from build123d import *
from build123d.topology import SkipClean

# Parameters (mm, degrees)
ESQUISSE1_W              = 55
ESQUISSE1_H              = 45
BOSS_EXTRU_1_DEPTH       = 12
ESQUISSE2_R              = 4.25
ENL_V_MAT_EXTRU_1_DEPTH  = 55.085580333
ESQUISSE3_R              = 7.75
ENL_V_MAT_EXTRU_2_DEPTH  = 12.25
ESQUISSE9_W              = 61.062756781
ESQUISSE9_H              = 12.22812859
ESQUISSE9_W_2            = 59.427147224
ESQUISSE9_H_2            = 8.100161614
ENL_V_MAT_EXTRU_7_DEPTH  = 31
SKETCH1_W                = 55
SKETCH1_H                = 36
BOSS_EXTRUDE1_DEPTH      = 5
SKETCH2_R                = 2.1
CUT_EXTRUDE1_DEPTH       = 38.003378224
SKETCH3_R                = 4
CUT_EXTRUDE2_DEPTH       = 10
CUT_EXTRUDE3_DEPTH       = 5
SKETCH5_R                = 2.1
CUT_EXTRUDE4_DEPTH       = 47.864165415
BOSS_EXTRUDE4_START      = 2
SKETCH7_R                = 2.1
BOSS_EXTRUDE4_DEPTH      = 2
SKETCH8_R                = 2.1
BOSS_EXTRUDE5_DEPTH      = 2
SKETCH9_W                = 7
SKETCH9_H                = 3.2
CUT_EXTRUDE6_DEPTH       = 8
SKETCH10_W               = 30
SKETCH10_H               = 15
BOSS_EXTRUDE6_DEPTH      = 90
BOSS_EXTRUDE7_DEPTH      = 5
BOSS_EXTRUDE7_DEPTH_BACK = 5


with BuildPart() as part:
    # Esquisse1 → Boss.-Extru.1 (new body)
    with BuildSketch(Plane.XY):
        Rectangle(ESQUISSE1_W, ESQUISSE1_H)
    extrude(amount=BOSS_EXTRU_1_DEPTH)

    # Esquisse2 → Enl_v. mat.-Extru.1 (cut, through all)
    with BuildSketch(Plane(origin=(0, 22.5, 0), x_dir=(1, 0, 0), z_dir=(0, 1, 0))):
        with Locations((-12.5, -12)):
            Circle(ESQUISSE2_R)
        with Locations((12.5, -12)):
            Circle(ESQUISSE2_R)
    extrude(amount=-ENL_V_MAT_EXTRU_1_DEPTH, mode=Mode.SUBTRACT)

    # Esquisse3 → Enl_v. mat.-Extru.2 (cut, symmetric)
    with BuildSketch(Plane(origin=(0, 0, 0), x_dir=(1, 0, 0), z_dir=(0, 1, 0))):
        with Locations((-12.5, -12)):
            Circle(ESQUISSE3_R)
    enl_v_mat_extru_2 = extrude(amount=ENL_V_MAT_EXTRU_2_DEPTH, both=True, mode=Mode.SUBTRACT)

    # Esquisse9 → Enl_v. mat.-Extru.7 (cut)
    with BuildSketch(Plane.XY.offset(12)):
        with Locations((-0.389430846, -24.114064295)):
            Rectangle(ESQUISSE9_W, ESQUISSE9_H)
        with Locations((1.674552641, 22.050080807)):
            Rectangle(ESQUISSE9_W_2, ESQUISSE9_H_2)
    extrude(amount=-ENL_V_MAT_EXTRU_7_DEPTH, mode=Mode.SUBTRACT)

    # Sketch1 → Boss-Extrude1 (add)
    with BuildSketch(Plane(origin=(0, 0, 0), x_dir=(-1, 0, 0), z_dir=(0, 0, -1))):
        Rectangle(SKETCH1_W, SKETCH1_H)
    extrude(amount=BOSS_EXTRUDE1_DEPTH)

    # Sketch2 → Cut-Extrude1 (cut, through all)
    with BuildSketch(Plane.XY.offset(12)):
        with Locations((-22.5, 13)):
            Circle(SKETCH2_R)
        with Locations(Location((22.5, 13, 0), (0, 0, 180))):
            Circle(SKETCH2_R)
        with Locations((22.5, -13)):
            Circle(SKETCH2_R)
        with Locations(Location((-22.5, -13, 0), (0, 0, 180))):
            Circle(SKETCH2_R)
    extrude(amount=-CUT_EXTRUDE1_DEPTH, mode=Mode.SUBTRACT)

    # Sketch3 → Cut-Extrude2 (cut)
    with BuildSketch(Plane(origin=(0, 0, -5), x_dir=(-1, 0, 0), z_dir=(0, 0, -1))):
        with Locations((-22.5, 13)):
            Circle(SKETCH3_R)
        with Locations((22.5, 13)):
            Circle(SKETCH3_R)
        with Locations((22.5, -13)):
            Circle(SKETCH3_R)
        with Locations((-22.5, -13)):
            Circle(SKETCH3_R)
    extrude(amount=-CUT_EXTRUDE2_DEPTH, mode=Mode.SUBTRACT)

    # Sketch4 → Cut-Extrude3 (cut)
    with BuildSketch(Plane(origin=(0, 0, -5), x_dir=(-1, 0, 0), z_dir=(0, 0, -1))):
        with BuildLine():
            Line((-18.5, 13), (-18.5, 18))
            Line((-18.5, 18), (-27.5, 18))
            Line((-27.5, 18), (-27.5, 9))
            Line((-27.5, 9), (-22.5, 9))
            ThreePointArc((-22.5, 9), (-25.328427125, 15.828427125), (-18.5, 13))
        make_face()
        with BuildLine():
            Line((-22.5, -9), (-27.5, -9))
            Line((-27.5, -9), (-27.5, -18))
            Line((-27.5, -18), (-18.5, -18))
            Line((-18.5, -18), (-18.5, -13))
            ThreePointArc((-18.5, -13), (-25.328427125, -15.828427125), (-22.5, -9))
        make_face()
        with BuildLine():
            Line((27.5, -18), (27.5, -9))
            Line((27.5, -9), (22.5, -9))
            ThreePointArc((22.5, -9), (25.328427125, -15.828427125), (18.5, -13))
            Line((18.5, -13), (18.5, -18))
            Line((18.5, -18), (27.5, -18))
        make_face()
        with BuildLine():
            Line((27.5, 18), (18.5, 18))
            Line((18.5, 18), (18.5, 13))
            ThreePointArc((18.5, 13), (25.328427125, 15.828427125), (22.5, 9))
            Line((22.5, 9), (27.5, 9))
            Line((27.5, 9), (27.5, 18))
        make_face()
    extrude(amount=-CUT_EXTRUDE3_DEPTH, mode=Mode.SUBTRACT)

    # Sketch5 → Cut-Extrude4 (cut, through all)
    with BuildSketch(Plane(origin=(0, 18, 0), x_dir=(1, 0, 0), z_dir=(0, 1, 0))):
        with Locations(Location((-10, 1, 0), (0, 0, 180))):
            Circle(SKETCH5_R)
        with Locations(Location((10, 1, 0), (0, 0, 180))):
            Circle(SKETCH5_R)
    extrude(amount=-CUT_EXTRUDE4_DEPTH, mode=Mode.SUBTRACT)

    # Sketch7 → Boss-Extrude4 (add)
    with SkipClean():  # the faces are left unmerged after this step: merging them gives an invalid solid
        with BuildSketch(Plane(origin=(0, 18, 0), x_dir=(1, 0, 0), z_dir=(0, 1, 0)).offset(BOSS_EXTRUDE4_START)):
            with BuildLine():
                Line((18.5, 5), (-18.5, 5))
                Line((-18.5, 5), (-18.5, 0))
                Line((-18.5, 0), (-27.5, 0))
                Line((-27.5, 0), (-27.5, -12))
                Line((-27.5, -12), (-16.75, -12))
                ThreePointArc((-16.75, -12), (-12.5, -7.75), (-8.25, -12))
                Line((-8.25, -12), (8.25, -12))
                ThreePointArc((8.25, -12), (12.5, -7.75), (16.75, -12))
                Line((16.75, -12), (27.5, -12))
                Line((27.5, -12), (27.5, 0))
                Line((27.5, 0), (18.5, 0))
                Line((18.5, 0), (18.5, 5))
            make_face()
            with Locations(Location((10, 1, 0), (0, 0, 180))):
                Circle(SKETCH7_R, mode=Mode.SUBTRACT)
            with Locations(Location((-10, 1, 0), (0, 0, 180))):
                Circle(SKETCH7_R, mode=Mode.SUBTRACT)
        extrude(amount=-BOSS_EXTRUDE4_DEPTH)
    add(part.part.scale(1), mode=Mode.REPLACE)  # the faces are merged on a copy

    # Sketch8 → Boss-Extrude5 (add)
    with BuildSketch(Plane.XZ.offset(18)):
        with BuildLine():
            Line((-27.5, 0), (-18.5, 0))
            Line((-18.5, 0), (-18.5, -5))
            Line((-18.5, -5), (18.5, -5))
            Line((18.5, -5), (18.5, 0))
            Line((18.5, 0), (27.5, 0))
            Line((27.5, 0), (27.5, 12))
            Line((27.5, 12), (16.75, 12))
            ThreePointArc((16.75, 12), (12.5, 7.75), (8.25, 12))
            Line((8.25, 12), (-8.25, 12))
            ThreePointArc((-8.25, 12), (-12.5, 7.75), (-16.75, 12))
            Line((-16.75, 12), (-27.5, 12))
            Line((-27.5, 12), (-27.5, 0))
        make_face()
        with Locations(Location((10, -1, 0), (0, 0, 180))):
            Circle(SKETCH8_R, mode=Mode.SUBTRACT)
        with Locations(Location((-10, -1, 0), (0, 0, 180))):
            Circle(SKETCH8_R, mode=Mode.SUBTRACT)
    extrude(amount=BOSS_EXTRUDE5_DEPTH)

    # Sketch9 → Cut-Extrude6 (cut)
    with BuildSketch(Plane(origin=(0, 0, -5), x_dir=(-1, 0, 0), z_dir=(0, 0, -1))):
        with Locations((-10, 14.4)):
            Rectangle(SKETCH9_W, SKETCH9_H)
        with Locations((10, 14.4)):
            Rectangle(SKETCH9_W, SKETCH9_H)
        with Locations((10, -14.4)):
            Rectangle(SKETCH9_W, SKETCH9_H)
        with Locations((-10, -14.4)):
            Rectangle(SKETCH9_W, SKETCH9_H)
    extrude(amount=-CUT_EXTRUDE6_DEPTH, mode=Mode.SUBTRACT)

    # Mirror1: Enl_v. mat.-Extru.2 across plane
    add(enl_v_mat_extru_2.mirror(Plane.ZY), mode=Mode.SUBTRACT)

    # Sketch10 → Boss-Extrude6 (add)
    with BuildSketch(Plane(origin=(0, 0, -5), x_dir=(-1, 0, 0), z_dir=(0, 0, -1))):
        Rectangle(SKETCH10_W, SKETCH10_H)
    extrude(amount=BOSS_EXTRUDE6_DEPTH)

    # Sketch11 → Boss-Extrude7 (add, two sides: drawn at the far end of the back side and taken through both)
    with BuildSketch(Plane.ZY.offset(-BOSS_EXTRUDE7_DEPTH_BACK)):
        Polygon((-5, 7.5), (-20.649753688, 7.5), (-5, 20), align=None)
    extrude(amount=BOSS_EXTRUDE7_DEPTH + BOSS_EXTRUDE7_DEPTH_BACK)


solid = part.part
Source: CAD feature listing. Evaluate the final solid. Frame: model axes, mm. A direction names the side the tool comes from. Give positions to 0.01 mm unless a question says otherwise; leave off trailing zeros. Order: outer loops, then holes, each group sorted by start corner. A loop starts at its lowest first (then second) coordinate and runs counter-clockwise, first axis right, second up. Notation, with made-up numbers: (83, 63) -> (112, 63) arc R7 ccw to (112, 72) -> close; hole circle Ø6 at (37.5, 43). An arc over 180 degrees is marked (long way). Use a Markdown table: item, result.
1) Section query D-D, the plane z = -17. Return the cut outline in (x, y), then the cut area to 3 significant figures.
Answer list:
| item | result |
|---|---|
| outline | (-15, -7.5) -> (15, -7.5) -> (15, 7.5) -> (5, 7.5) -> (5, 10.42) -> (-5, 10.42) -> (-5, 7.5) -> (-15, 7.5) -> close |
| area | 479 mm² |
2) Contact query for flat-ended pins moving along their axis: P1, Ø3.5, axis at x = -9.5, z = 0, coming from the +Y side; P2, Ø10, axis at x = 12.5, z = -75, coming from the +Y side; P3, Ø5.5, axis at x = -22.5, y = -13, coming from the -Z side; P4, Ø1.6, axis at x = 9, y = -14, coming from the -Z side. Output: stop coordinate, or through.
Answer list:
| item | result |
|---|---|
| P1 | y = 20 |
| P2 | y = 7.5 |
| P3 | z = 5 |
| P4 | z = 3 |
3) Section query C-C, the plane z = -61. Return the cut outline in (x, y), then the cut area to 3 significant figures.
Answer list:
| item | result |
|---|---|
| outline | (-15, -7.5) -> (15, -7.5) -> (15, 7.5) -> (-15, 7.5) -> close |
| area | 450 mm² |
4) Ray query, line 1 along Y through (x, z) = (22.5, 9.25); line 2 along Z through (x, y) = (17, -14.5); line 3 along X through (y, z) = (-4, -30). Return the intervals inside material, ascending. Write a range as [from, to].
Answer list:
| item | result |
|---|---|
| line 1 | [-20, -15.1], [-10.9, 10.9], [15.1, 20] |
| line 2 | [-5, 12] |
| line 3 | [-15, 15] |
5) Section query B-B, the plane x = 10. Count the separate pieces of the cut face and the enclosed holes in it, then the cut area to 3 significant figures.
Answer list:
| item | result |
|---|---|
| separate pieces | 4 |
| enclosed holes | 0 |
| area | 1,600 mm² |
6) Reachability of faces 4 (the flat face through (0, -7.5, -49)), 5 (the flat face through (24, 17, 0)), 6 (the flat face through (-13.5, -14, -1)) from +Z, -Z, +X, -X, +Y, -Y: full face, straight path, thin tool, end or side. Return the list, or none.
Answer list:
| item | result |
|---|---|
| face 4 | -Z, +X, -X, -Y |
| face 5 | -Z, +X, +Y |
| face 6 | -Z |
7) Mould query, pull axis X, two halves, no side actions, for faces 1 (the flat face through (0, 7.5, -49)), 2 (the flat face through (-18.5, -16, -2)), 3 (the cylindrical face through (-7.9, -17.97, -1.09)). Classes: +X half, -X half, draft (parallel to the pull), parting line (faces both ways), or undercut.
Answer list:
| item | result |
|---|---|
| face 1 | draft |
| face 2 | -X half |
| face 3 | undercut |
8) Section query A-A, the plane y = 4.5. Return the cut outline in (x, z), then the cut area to 3 significant figures.
Answer list:
| item | result |
|---|---|
| outline | (-27.5, -5) -> (-15, -5) -> (-15, -95) -> (15, -95) -> (15, -5) -> (27.5, -5) -> (27.5, 12) -> (20.25, 12) arc R7.75 cw to (4.75, 12) -> (-4.75, 12) arc R7.75 cw to (-20.25, 12) -> (-27.5, 12) -> close; hole circle Ø4.2 at (-10, -1); hole circle Ø4.2 at (10, -1) |
| area | 3,420 mm² |
